Here's how the part is built. I have some questions about the finished solid (model axes, mm). A direction names the side the tool comes from. Round coordinates to 2 decimals unless told otherwise and drop trailing zeros. Write each loop counter-clockwise with the first axis right and the second up, starting at its lowest first coordinate (ties: lowest second). Pieces come first, ordered by that corner, then holes. Notation, with made-up numbers: (6, 29) -> (18, 29) arc R31 ccw to (18, 60) -> close; hole circle Ø1 at (-33.75, 25.25). An arc over 180 degrees is marked (long way). Put each result on its own line as item: value. Start each with the question number.
1. Suppose I cut it at A-A (z = 6.75). Please give me the cut outline in (x, y), then the cut area to 3 significant figures.
2. Which directions (+Z, -Z, +X, -X, +Y, -Y) give clear straight access to the entire face, cutting with the end or side of a thin tool? Please do faces 1 (the face through (14, 21, 29)), 2 (the face through (0, 12, 15)), 3 (the face through (13, 21.5, 11)), 4 (the face through (5, 10, 14)).
3. For pin 1 (8 mm diameter, centred on x = 7.5, y = 5.5, fed in from +Z); pin 2 (8 mm diameter, centred on y = 3.5, z = 10, fed in from +X); pin 3 (8 mm diameter, centred on x = 22, z = 17, fed in from -Y), each with a flat end and sliding along its axis, tell me the tip position at first contact or that it passes through.
4. We'd pull the mould along X, two halves only. Please class faces 5 (the face through (25, 23, 15)), 6 (the face through (12, 23.5, 11)), 7 (the face through (3, 16, 22)), 8 (the face through (2, 0, 15)): +X half, -X half, draft (parallel to the pull), parting line (faces both ways), or undercut.
5. Suppose I cut it at D-D (z = 23.5). Please give me the cut outline in (x, y), then the cut area to 3 significant figures.
6. I need wall thicknesses on probe 1 along Y at (x, z) = (13.25, 20); probe 2 along X at (y, z) = (3.75, 20.25); probe 3 along Y at (x, z) = (3.25, 11.75). Which ranges of each line are inside material? Lowest first, please. Write a range as from..to.
7. Suppose I cut it at B-B (x = 4.25). Please give me the cut outline in (y, z).
8. Suppose I cut it at C-C (y = 10.5). Please give me the cut outline in (x, z).
Autodesk Fusion 360 part; units mm, degrees
sketch "Sketch1" plane through (0, 0, 0) normal (0, 0, 1) x (1, 0, 0)
  line L0 (0, 0) -> (0, 25)
  line L1 (0, 25) -> (25, 25)
  line L2 (25, 25) -> (25, 20)
  line L3 (0, 0) -> (5, 0)
  line L4 (5, 0) -> (5, 20)
  line L5 (5, 20) -> (25, 20)
  dimension "d5" = 25
  dimension "d6" = 25
  dimension "d7" = 5
  dimension "d8" = 5
extrude "Extrude1" add sketch "Sketch1" along normal blind 30
chamfer "Chamfer1" distance 2 angle 45 1 edges at (5, 10, 30)
chamfer "Chamfer2" distance 2 angle 45 1 edges at (14, 20, 30)
sketch "Sketch2" plane through (0, 0, 0) normal (0, 0, -1) x (1, 0, 0)
  line L0 (5, 0) -> (0, 0)
  line L1 (0, 0) -> (0, -25)
  line L2 (0, -25) -> (25, -25)
  line L3 (25, -25) -> (25, -20)
  line L4 (25, -20) -> (5, -20)
  line L5 (5, -20) -> (5, 0)
  line L6 (1.5, -2) -> (3.5, -2)
  line L7 (1.5, -21.5) -> (1.5, -23.5)
  line L8 (23, -21.5) -> (23, -23.5)
  line L9 (3.5, -2) -> (3.5, -21.5)
  line L10 (1.5, -2) -> (1.5, -21.5)
  line L11 (23, -21.5) -> (3.5, -21.5)
  line L12 (23, -23.5) -> (1.5, -23.5)
  dimension "d13" = 2
  dimension "d14" = 1.5
  dimension "d18" = 1.5
  dimension "d19" = 2
  dimension "d20" = 2
  dimension "d21" = 2
extrude "Extrude2" cut sketch "Sketch2" against normal blind 22 contours L6 L7 L8 L9 L10 L11 L12
Verdict:
1. outline: (0, 0) -> (5, 0) -> (5, 20) -> (25, 20) -> (25, 25) -> (0, 25) -> close; hole (1.5, 2) -> (3.5, 2) -> (3.5, 21.5) -> (23, 21.5) -> (23, 23.5) -> (1.5, 23.5) -> close
1. area: 143 mm^2
2. face 1: +Z, +X, -Y
2. face 2: +Z, -Z, -X, +Y, -Y
2. face 3: -Z
2. face 4: +Z, -Z, +X, -Y
3. pin 1: stops at z = 29.5
3. pin 2: stops at x = 5
3. pin 3: stops at y = 20
4. face 5: +X half
4. face 6: undercut
4. face 7: undercut
4. face 8: draft
5. outline: (0, 0) -> (5, 0) -> (5, 20) -> (25, 20) -> (25, 25) -> (0, 25) -> close
5. area: 225 mm^2
6. probe 1: y = 20..21.5, 23.5..25
6. probe 2: x = 0..1.5, 3.5..5
6. probe 3: y = 0..2, 23.5..25
7. outline: (0, 0) -> (21.5, 0) -> (21.5, 22) -> (23.5, 22) -> (23.5, 0) -> (25, 0) -> (25, 30) -> (22, 30) -> (20.75, 28.75) -> (0, 28.75) -> close
8. outline: (0, 0) -> (1.5, 0) -> (1.5, 22) -> (3.5, 22) -> (3.5, 0) -> (5, 0) -> (5, 28) -> (3, 30) -> (0, 30) -> close
